from build123d import *

# Parameters (mm, degrees)
SKETCH1_W           = 217
SKETCH1_H           = 127
BOSS_EXTRUDE1_DEPTH = 95
SKETCH2_R           = 5
BOSS_EXTRUDE2_DEPTH = 40
SKETCH3_R           = 12.5
BOSS_EXTRUDE3_DEPTH = 20


with BuildPart() as part:
    # Sketch1 → Boss-Extrude1 (new body)
    with BuildSketch(Plane(origin=(0, 0, 0), x_dir=(1, 0, 0), z_dir=(0, 1, 0))):
        Rectangle(SKETCH1_W, SKETCH1_H)
    extrude(amount=BOSS_EXTRUDE1_DEPTH)

    # Sketch2 → Boss-Extrude2 (add)
    with BuildSketch(Plane(origin=(0, 95, 0), x_dir=(1, 0, 0), z_dir=(0, 1, 0))):
        with Locations((-58.5, 23.5)):
            Circle(SKETCH2_R)
        with Locations((58.5, 23.5)):
            Circle(SKETCH2_R)
    extrude(amount=BOSS_EXTRUDE2_DEPTH)

    # Sketch3 → Boss-Extrude3 (add)
    with BuildSketch(Plane(origin=(0, 135, 0), x_dir=(1, 0, 0), z_dir=(0, 1, 0))):
        with Locations((-58.5, 23.5)):
            Circle(SKETCH3_R)
        with Locations((58.5, 23.5)):
            Circle(SKETCH3_R)
    extrude(amount=BOSS_EXTRUDE3_DEPTH)


solid = part.part
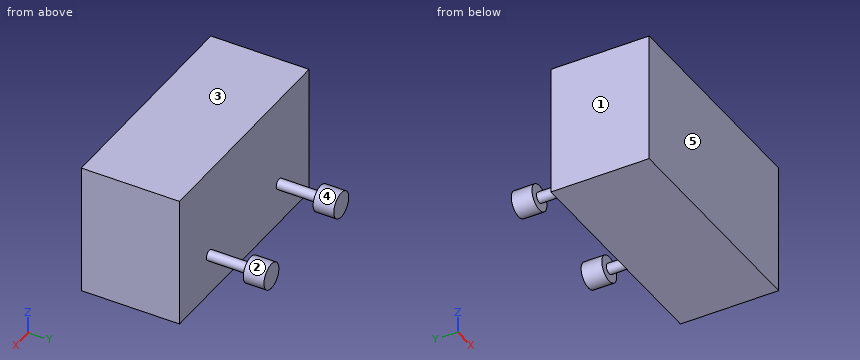
Geometry: final body of the model. Coordinates: model frame, mm. Face numbers are marked on the shaded views. A direction names the side the tool comes from. Give positions to 0.01 mm unless a question says otherwise; leave off trailing zeros. Write each loop counter-clockwise with the first axis right and the second up, starting at its lowest first coordinate (ties: lowest second). Pieces come first, ordered by that corner, then holes. Notation, with made-up numbers: (-0.5, -36) -> (53.5, -36) arc R23 cw to (53.5, -1) -> close; hole circle Ø5 at (-37, 34.5). An arc over 180 degrees is marked (long way). Answer in a Markdown table with one row per item.
(1) Section query C-C on y = 108.5. Return loops of the section in (x, z).
Answers below:
| item | result |
|---|---|
| outline | circle Ø10 at (-58.5, -23.5); circle Ø10 at (58.5, -23.5) |
(2) Ray query, line 1 along Y through (x, z) = (83.5, -50.5); line 2 along Z through (x, y) = (61.5, 133.5). Return the intervals inside material, ascending. Write a range as [from, to].
Answers below:
| item | result |
|---|---|
| line 1 | [0, 95] |
| line 2 | [-27.5, -19.5] |
(3) Section query D-D on z = 45.5. Return loops of the section in (x, y).
Answers below:
| item | result |
|---|---|
| outline | (-108.5, 0) -> (108.5, 0) -> (108.5, 95) -> (-108.5, 95) -> close |
(4) Section query A-A on z = -23.5. Return loops of the section in (x, y).
Answers below:
| item | result |
|---|---|
| outline | (-108.5, 0) -> (108.5, 0) -> (108.5, 95) -> (63.5, 95) -> (63.5, 135) -> (71, 135) -> (71, 155) -> (46, 155) -> (46, 135) -> (53.5, 135) -> (53.5, 95) -> (-53.5, 95) -> (-53.5, 135) -> (-46, 135) -> (-46, 155) -> (-71, 155) -> (-71, 135) -> (-63.5, 135) -> (-63.5, 95) -> (-108.5, 95) -> close |
(5) Section query B-B on x = 58.5. Return loops of the section in (y, z).
Answers below:
| item | result |
|---|---|
| outline | (0, -63.5) -> (95, -63.5) -> (95, -28.5) -> (135, -28.5) -> (135, -36) -> (155, -36) -> (155, -11) -> (135, -11) -> (135, -18.5) -> (95, -18.5) -> (95, 63.5) -> (0, 63.5) -> close |
(6) Draft query along X for the marked faces 1, 2 and 3. Return one class per face: +X half, -X half, draft (parallel to the pull), parting line (faces both ways), or undercut.
Answers below:
| item | result |
|---|---|
| face 1 | -X half |
| face 2 | undercut |
| face 3 | draft |
(7) Set-up query: the marked faces 4 and 5. Return all of +Z, -Z, +X, -X, +Y, -Y with unobstructed straight access to the full face (end or side cutting, diameter ignored); none if empty.
Answers below:
| item | result |
|---|---|
| face 4 | +Y |
| face 5 | +Z, -Z, +X, -X, -Y |
